Source: CAD feature listing. Evaluate the final solid. Frame: model axes, mm. Face numbers are marked on the shaded views. A direction names the side the tool comes from. Give positions to 0.01 mm unless a question says otherwise; leave off trailing zeros. Write each loop counter-clockwise with the first axis right and the second up, starting at its lowest first coordinate (ties: lowest second). Pieces come first, ordered by that corner, then holes. Notation, with made-up numbers: (-1, 26.25) -> (36, 26.25) arc R20 ccw to (36, 53.25) -> close; hole circle Ø3 at (-31.75, 77). An arc over 180 degrees is marked (long way). Write item = value, one per line.
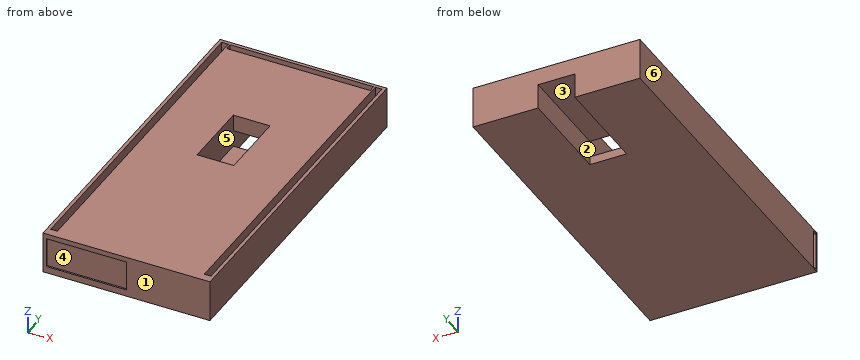
Autodesk Fusion 360 part; units mm, degrees
sketch "Sketch1" plane through (0, 0, 0) normal (0, 0, 1) x (1, 0, 0)
  line L0 (-50, 100) -> (0, 100)
  line L1 (0, 100) -> (0, -2.5)
  line L2 (0, -2.5) -> (-50, -2.5)
  line L3 (-50, -2.5) -> (-50, 100)
  dimension "d1" = 50
  dimension "d2" = 102.5
extrude "Extrude1" add sketch "Sketch1" along normal blind 12.5
sketch "Sketch2" plane through (0, 0, 12.5) normal (0, 0, 1) x (-1, 0, 0)
  line L0 (50, 2.5) -> (0, 2.5)
  line L1 (0, 2.5) -> (0, -100)
  line L2 (0, -100) -> (50, -100)
  line L3 (50, -100) -> (50, 2.5)
  line L4 (50, -100) -> (49, -100)
  line L5 (49, -100) -> (49, -99)
  line L6 (49, -99) -> (47, -99)
  line L7 (47, -99) -> (47, 0)
  line L8 (47, 0) -> (49, 0)
  line L9 (49, 0) -> (49, -99)
  line L10 (50, -100) -> (0, -100)
  line L11 (3, -99) -> (3, 0)
  line L12 (1, 0) -> (1, -99)
  line L13 (1, -99) -> (3, -99)
  line L14 (3, 0) -> (1, 0)
  line L15 (47, -99) -> (46.5, -99)
  line L16 (46.5, -99) -> (3.5, -99)
  line L17 (3.5, -99) -> (3.5, -97)
  line L18 (3.5, -97) -> (46.5, -97)
  line L19 (46.5, -97) -> (46.5, -99)
  dimension "d5" = 2
  dimension "d6" = 99
  dimension "d7" = 43
  dimension "d8" = 2
extrude "Extrude2" cut sketch "Sketch2" against normal blind 3 contours L16 L17 L18 L19 | L6 L7 L8 L9 | L11 L12 L13 L14
sketch "Sketch3" plane through (0, 0, 12.5) normal (0, 0, 1) x (-1, 0, 0)
  line L0 (47, -99) -> (47, 0)
  line L1 (47, 0) -> (49, 0)
  line L2 (49, 0) -> (49, -99)
  line L3 (49, -99) -> (47, -99)
  line L4 (1, -99) -> (1, 0)
  line L5 (1, 0) -> (3, 0)
  line L6 (3, 0) -> (3, -99)
  line L7 (3, -99) -> (1, -99)
  line L8 (3.5, -99) -> (3.5, -97)
  line L9 (3.5, -97) -> (46.5, -97)
  line L10 (46.5, -97) -> (46.5, -99)
  line L11 (46.5, -99) -> (3.5, -99)
  line L12 (50, 2.5) -> (0, 2.5)
  line L13 (0, 2.5) -> (0, -100)
  line L14 (0, -100) -> (50, -100)
  line L15 (50, -100) -> (50, 2.5)
  line L16 (50, -100) -> (50, -70)
  line L17 (50, -70) -> (30.5, -70)
  line L18 (30.5, -70) -> (19.5, -70)
  line L19 (19.5, -70) -> (19.5, -49)
  line L20 (19.5, -49) -> (30.5, -49)
  line L21 (30.5, -49) -> (30.5, -70)
  dimension "d11" = 30
  dimension "d12" = 19.5
  dimension "d13" = 11
  dimension "d14" = 21
extrude "Extrude3" cut sketch "Sketch3" against normal blind 10 contours L18 L19 L20 L21
sketch "Sketch4" plane through (0, 0, 2.5) normal (0, 0, 1) x (-1, 0, 0)
  line L0 (30.5, -49) -> (19.5, -49)
  line L1 (19.5, -49) -> (19.5, -70)
  line L2 (19.5, -70) -> (30.5, -70)
  line L3 (30.5, -70) -> (30.5, -49)
  line L4 (30.5, -67.3616) -> (19.5, -67.3616)
  line L5 (19.5, -67.3616) -> (19.5, -100.8789)
  line L6 (19.5, -100.8789) -> (30.5, -100.8789)
  line L7 (30.5, -100.8789) -> (30.5, -67.3616)
extrude "Extrude4" cut sketch "Sketch4" against normal blind 30 contours L2 L5 L6 L7
extrude "Extrude5" cut 1 faces at (-26.8333, 90, 2.5) along direction (0, 0, 1) blind 5
sketch "Sketch5" plane through (-50, 0, 0) normal (-1, 0, 0) x (0, -1, 0)
  line L0 (-100, 0) -> (2.5, 0)
  line L1 (2.5, 0) -> (2.5, 12.5)
  line L2 (2.5, 12.5) -> (-100, 12.5)
  line L3 (-100, 12.5) -> (-100, 0)
  line L4 (2.5, 0) -> (2.5, 2)
  line L5 (2.5, 2) -> (2, 2)
  line L6 (2, 2) -> (2, 11)
  line L7 (2, 11) -> (2.5, 11)
  line L8 (2, 11) -> (2, 12)
  line L9 (2, 12) -> (0.5, 12)
  line L10 (0.5, 12) -> (0.5, 0.4)
  line L11 (0.5, 0.4) -> (2, 0.4)
  line L12 (2, 0.4) -> (2, 2)
  dimension "d21" = 1.5
  dimension "d22" = 11.6
extrude "Extrude6" cut sketch "Sketch5" against normal blind 30 contours L6 L8 L9 L10 L11 L12
extrude "Extrude7" cut sketch "Sketch5" against normal blind 25 contours L1 L5 L6 L7
extrude "Extrude8" add sketch "Sketch5" against normal blind 1 contours L1 L5 L6 L7
1) Material intervals for L1, parallel to X at y = 96, z = 10.75; L2, parallel to Y at x = -24.5, z = 2; L3, parallel to X at y = 62.5, z = 9.25, sorted ascending.
Computed:
L1 = -50 to -49, -47 to -3, -1 to 0
L2 = -2.5 to -2, -0.5 to 70
L3 = -50 to -30.5, -19.5 to 0
2) Cut plane C-C (y = 65). Return the cut outline in (x, z), then the cut area to 3 significant figures.
Computed:
outline = (-50, 0) -> (0, 0) -> (0, 12.5) -> (-1, 12.5) -> (-1, 9.5) -> (-3, 9.5) -> (-3, 12.5) -> (-19.5, 12.5) -> (-19.5, 2.5) -> (-30.5, 2.5) -> (-30.5, 12.5) -> (-47, 12.5) -> (-47, 9.5) -> (-49, 9.5) -> (-49, 12.5) -> (-50, 12.5) -> close
area = 503 mm²
3) Contact query for flat-ended pins moving along their axis: pin 1 (1.2 mm diameter, centred on x = -25.5, z = 1.5, fed in from +Y); pin 2 (1 mm diameter, centred on x = -48, y = 34, fed in from +Z); pin 3 (5.5 mm diameter, centred on x = -23.5, y = 56.5, fed in from +Z). Output: stop coordinate, or through.
Computed:
pin_1 = 70
pin_2 = 9.5
pin_3 = 2.5
4) Draft query along Y for the marked faces 1, 2, 3 and 4. Return one class per face: pulls with the +Y half, pulls with the -Y half, needs draft (parallel to the pull), parting line crosses it, or undercut.
Computed:
face_1 = pulls with the -Y half
face_2 = undercut
face_3 = needs draft
face_4 = undercut
5) Access query for the marked faces 5 and 6. Directions: +Z, -Z, +X, -X, +Y, -Y. A direction counts if a zero-diameter tool reaches every point of the face in a straight line with its end or side. Return the directions, or none.
Computed:
face_5 = none
face_6 = +Z, -Z, -X, +Y, -Y
6) Cut plane B-B (x = -38.5). Return the cut outline in (y, z).
Computed:
outline = (-2.5, 0) -> (100, 0) -> (100, 12.5) -> (99, 12.5) -> (99, 9.5) -> (97, 9.5) -> (97, 12.5) -> (-2.5, 12.5) -> (-2.5, 11) -> (-2, 11) -> (-2, 12) -> (-0.5, 12) -> (-0.5, 0.4) -> (-2, 0.4) -> (-2, 2) -> (-2.5, 2) -> close
7) Cut plane A-A (z = 8.5). Return the cut outline in (x, y).
Computed:
outline = (-50, -2.5) -> (-49, -2.5) -> (-49, -2) -> (-50, -2) -> close; (-50, -0.5) -> (-20, -0.5) -> (-20, -2) -> (-25, -2) -> (-25, -2.5) -> (0, -2.5) -> (0, 100) -> (-50, 100) -> close; hole (-30.5, 49) -> (-19.5, 49) -> (-19.5, 70) -> (-30.5, 70) -> close
8) Cut plane D-D (y = 30). Return the cut outline in (x, z).
Computed:
outline = (-50, 0) -> (0, 0) -> (0, 12.5) -> (-1, 12.5) -> (-1, 9.5) -> (-3, 9.5) -> (-3, 12.5) -> (-47, 12.5) -> (-47, 9.5) -> (-49, 9.5) -> (-49, 12.5) -> (-50, 12.5) -> close
